Read the model definition and answer for the solid it produces. Units are mm, in the model's axes. A direction names the side the tool comes from. Coordinates: 2 decimals unless noted, no trailing zeros. Order: outer loops, then holes, each group sorted by start corner. A loop starts at its lowest first (then second) coordinate and runs counter-clockwise, first axis right, second up. Notation, with made-up numbers: (60.5, -26.5) -> (97.5, -26.5) arc R13 ccw to (97.5, -16.5) -> close; hole circle Ø6 at (-5.75, 10.25). An arc over 180 degrees is marked (long way). Use CSV: the item, a comma, the result in double quotes.
```python
from build123d import *

# Parameters (mm, degrees)
REDONDEO1_R                   = 2.5
TALADRO_ROSCADO_M3X0_51_D     = 2.5
TALADRO_ROSCADO_M3X0_51_DEPTH = 8.5
TALADRO_ROSCADO_M3X0_51_TIP   = 0.751075774
CHAFL_N1_SIZE                 = 0.5


with BuildPart() as part:
    # Croquis1 → Revolución1 (revolve)
    with BuildSketch(Plane(origin=(0, 0, 0), x_dir=(0, 1, 0), z_dir=(0, 0, 1)), mode=Mode.PRIVATE) as revoluci_n1_sk:
        Polygon((0, 0), (1.5, 0), (1.5, 6.25), (5, 6.25), (5, 9.25), (16, 9.25), (16, 56.25), (5, 56.25), (5, 59.85), (1.6, 59.85), (1.6, 67), (0, 67), align=None)
    revolve(revoluci_n1_sk.sketch.rotate(Axis((0, 0, 0), (-1, 0, 0)), 90), axis=Axis((0, 0, 0), (-1, 0, 0)))

    # Redondeo1
    redondeo1_edges = [part.edges().sort_by_distance(p)[0] for p in [
        (-56.25, 0, 16),
    ]]
    fillet(redondeo1_edges, radius=REDONDEO1_R)

    # Taladro roscado M3x0.51
    with Locations(Plane(origin=(-56.25, 0, 0), x_dir=(0, -1, 0), z_dir=(-1, 0, 0))):
        with Locations((-10.3, 0), (10.3, 0)):
            Hole(TALADRO_ROSCADO_M3X0_51_D / 2, depth=TALADRO_ROSCADO_M3X0_51_DEPTH)
            with Locations((0, 0, -(TALADRO_ROSCADO_M3X0_51_DEPTH + TALADRO_ROSCADO_M3X0_51_TIP / 2))):  # 118° drill point
                Cone(0, TALADRO_ROSCADO_M3X0_51_D / 2, TALADRO_ROSCADO_M3X0_51_TIP, mode=Mode.SUBTRACT)

    # Chaflán1
    chafl_n1_edges = [part.edges().sort_by_distance(p)[0] for p in [
        (-67, 0, 1.6),
    ]]
    chamfer(chafl_n1_edges, length=CHAFL_N1_SIZE)


solid = part.part
```
Item 1: Find section B-B, the plane x = -62. Give the vertices of the cut face in (y, z), then the cut area to 3 significant figures.
Return value:
outline,"circle Ø3.2 at (0, 0)"
area,"8.04 mm^2"
Item 2: The mould has two halves that part along Y. Classify faces 1 (the flat face through (-56.25, 6, 0)), 2 (the conical face through (-47.129, -10.128, -0.132)), 3 (the cylindrical face through (-63.222, -0.481, -1.526)), 4 (the cylindrical face through (-51.94, -9.145, -0.479)): +Y half, -Y half, draft (parallel to the pull), parting line (faces both ways), or undercut.
Return value:
face 1,"draft"
face 2,"undercut"
face 3,"parting line"
face 4,"undercut"
Item 3: Each of these flat-tipped pins is pushed along its axis until it touches: P1, Ø8, axis at y = -4.5, z = 6.5, coming from the -X side; P2, Ø10, axis at x = -16.5, y = -6.5, coming from the +Z side; P3, Ø5, axis at y = -0.5, z = -10, coming from the +X side; P4, Ø8, axis at y = -1.5, z = -2, coming from the -X side. Where does it stop, or does it pass through?
Return value:
P1,"stops at x = -59.85"
P2,"stops at z = 15.93"
P3,"stops at x = -9.25"
P4,"stops at x = -67"
Item 4: Straight lines are drawn through the part: line 1 along Y through (x, z) = (-51.25, 0); line 2 along Y through (x, z) = (-56, -0.5); line 3 along X through (y, z) = (-10.5, 8.5). For each, find the intervals that lie inside material, in ascending order.
Return value:
line 1,"y = -16 to -11.55, -9.05 to 9.05, 11.55 to 16"
line 2,"y = -14.58 to -11.45, -9.15 to 9.15, 11.45 to 14.58"
line 3,"x = -56.25 to -9.25"
Item 5: Find section C-C, the plane x = -31. Give the vertices of the cut face in (y, z), then the cut area to 3 significant figures.
Return value:
outline,"circle Ø32 at (0, 0)"
area,"804 mm^2"
Item 6: A tool of negligible diameter and unlimited length cuts with its end or side. For faces 5 (the cylindrical face through (-51.94, 9.05, 0.05)), 6 (the cylindrical face through (-31.81, 15.62, 3.47)), 7 (the cylindrical face through (-8, 0, 5)), from which of +Z, -Z, +X, -X, +Y, -Y can it reach the whole face along a straight path? Write none if from no direction.
Return value:
face 5,"-X"
face 6,"+X, -X"
face 7,"+X"
Item 7: Find section A-A, the plane y = 0. Give the vertices of the cut face in (x, z).
Return value:
outline,"(-67, -1.1) -> (-66.5, -1.6) -> (-59.85, -1.6) -> (-59.85, -5) -> (-56.25, -5) -> (-56.25, -13.5) arc R2.5 ccw to (-53.75, -16) -> (-9.25, -16) -> (-9.25, -5) -> (-6.25, -5) -> (-6.25, -1.5) -> (0, -1.5) -> (0, 1.5) -> (-6.25, 1.5) -> (-6.25, 5) -> (-9.25, 5) -> (-9.25, 16) -> (-53.75, 16) arc R2.5 ccw to (-56.25, 13.5) -> (-56.25, 5) -> (-59.85, 5) -> (-59.85, 1.6) -> (-66.5, 1.6) -> (-67, 1.1) -> close"
